Verification items for this drawing (mm, ordinates from the low corner). A direction names the side the tool comes from. Round coordinates to 2 decimals unless told otherwise and drop trailing zeros. Loops run counter-clockwise (first coordinate to the right, second up) from the corner with the lowest first, then second, coordinate; pieces in that order, holes last. Notation, with made-up numbers: (32, 68) - (59, 68) arc R34 cw to (59, 105) - close; hole circle Ø4 at (19.5, 47.25). An arc over 180 degrees is marked (long way). Put each result on its own line as item: value. Start each with the question number.
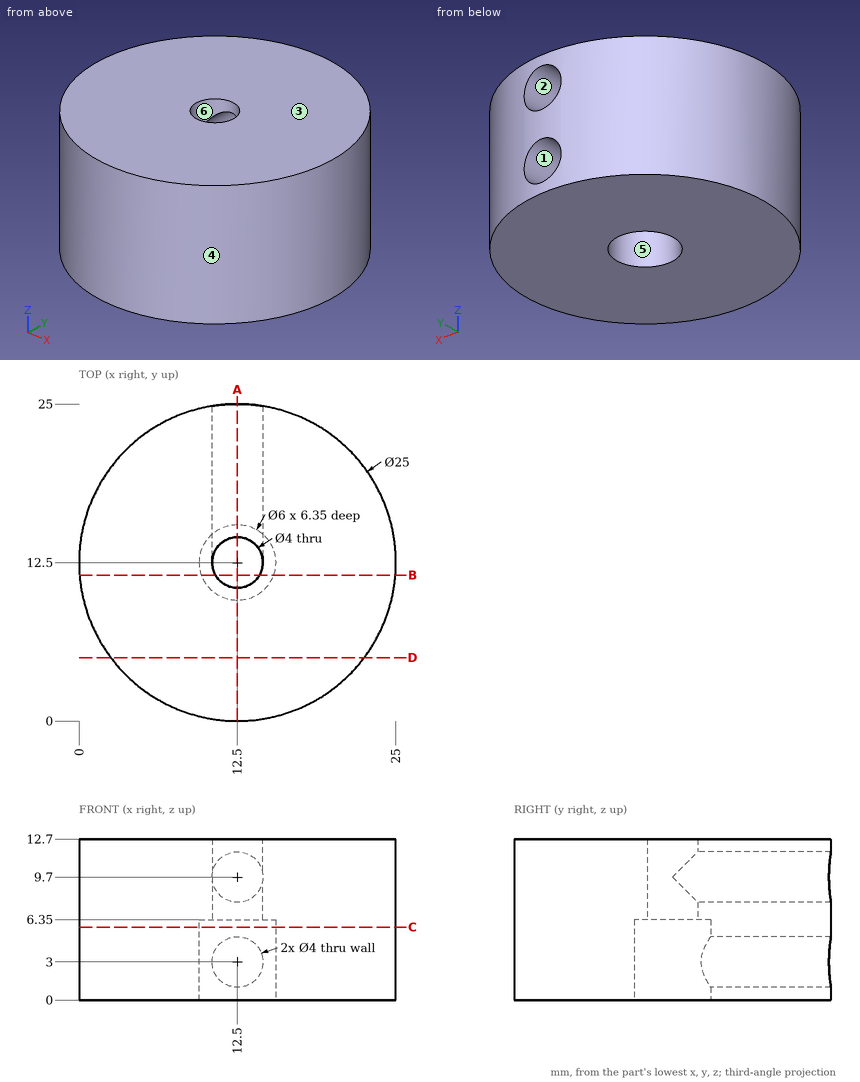
Q1. Cross-section at D-D on y = 5. Enter the section's corners in (x, z), and give its area (3 significant figures).
Q2. Material ranges on line 1 (Z direction, x = 12.5, y = 23.25); line 2 (Z direction, x = 13, y = 16); line 3 (Y direction, x = 12.5, z = 3), recorded low to high. Write a range as from..to.
Q3. Cross-section at C-C on z = 5.75. Enter the section's corners in (x, y), and give its area (3 significant figures).
Q4. Draft check along X on the marked faces 1, 2, 3 and 4. Enter one of: +X half, -X half, draft (parallel to the pull), parting line (faces both ways), or undercut.
Q5. Cross-section at B-B on y = 11.5. Enter the section's corners in (x, z), and give its area (3 significant figures).
Q6. Cross-section at A-A on x = 12.5. Enter the section's corners in (y, z), and give its area (3 significant figures).
Q7. Set-up check for the marked faces 5 and 6: record each of +Z, -Z, +X, -X, +Y, -Y from which the full face is reachable in a straight line by a thin tool's end or side.
Q8. Depth check by flat-ended pin: pin 1 Ø5 at (x, y) = (12.5, 12.5) entering from -Z; pin 2 Ø6 at (x, z) = (18, 1.5) entering from +Y; pin 3 Ø2 at (x, z) = (4.5, 7.5) entering from +Y; pin 4 Ø5 at (x, y) = (13.5, 13.5) entering from -Z. Enter the tip coordinate at first touch or a pass-through.
Answer list:
1. outline: (2.5, 0) - (22.5, 0) - (22.5, 12.7) - (2.5, 12.7) - close
1. area: 254 mm2
2. line 1: z = 0..1, 5..7.7, 11.7..12.7
2. line 2: z = 0..1.06, 4.94..7.76, 11.64..12.7
2. line 3: y = 0..9.5
3. outline: circle Ø25 at (12.5, 12.5); hole circle Ø6 at (12.5, 12.5)
3. area: 463 mm2
4. face 1: undercut
4. face 2: undercut
4. face 3: draft
4. face 4: parting line
5. outline: (0.04, 0) - (9.67, 0) - (9.67, 6.35) - (10.77, 6.35) - (10.77, 12.7) - (0.04, 12.7) - close; (14.23, 6.35) - (15.33, 6.35) - (15.33, 0) - (24.96, 0) - (24.96, 12.7) - (14.23, 12.7) - close
5. area: 259 mm2
6. outline: (0, 0) - (9.5, 0) - (9.5, 6.35) - (10.5, 6.35) - (10.5, 12.7) - (0, 12.7) - close; (14.5, 6.35) - (15.5, 6.35) - (15.5, 5) - (25, 5) - (25, 7.7) - (14.5, 7.7) - close; (14.5, 11.7) - (25, 11.7) - (25, 12.7) - (14.5, 12.7) - close; (15.5, 0) - (25, 0) - (25, 1) - (15.5, 1) - close
6. area: 174 mm2
7. face 5: -Z
7. face 6: +Z, -Z
8. pin 1: stops at z = 6.35
8. pin 2: stops at y = 24.75
8. pin 3: stops at y = 22.86
8. pin 4: stops at z = 0
